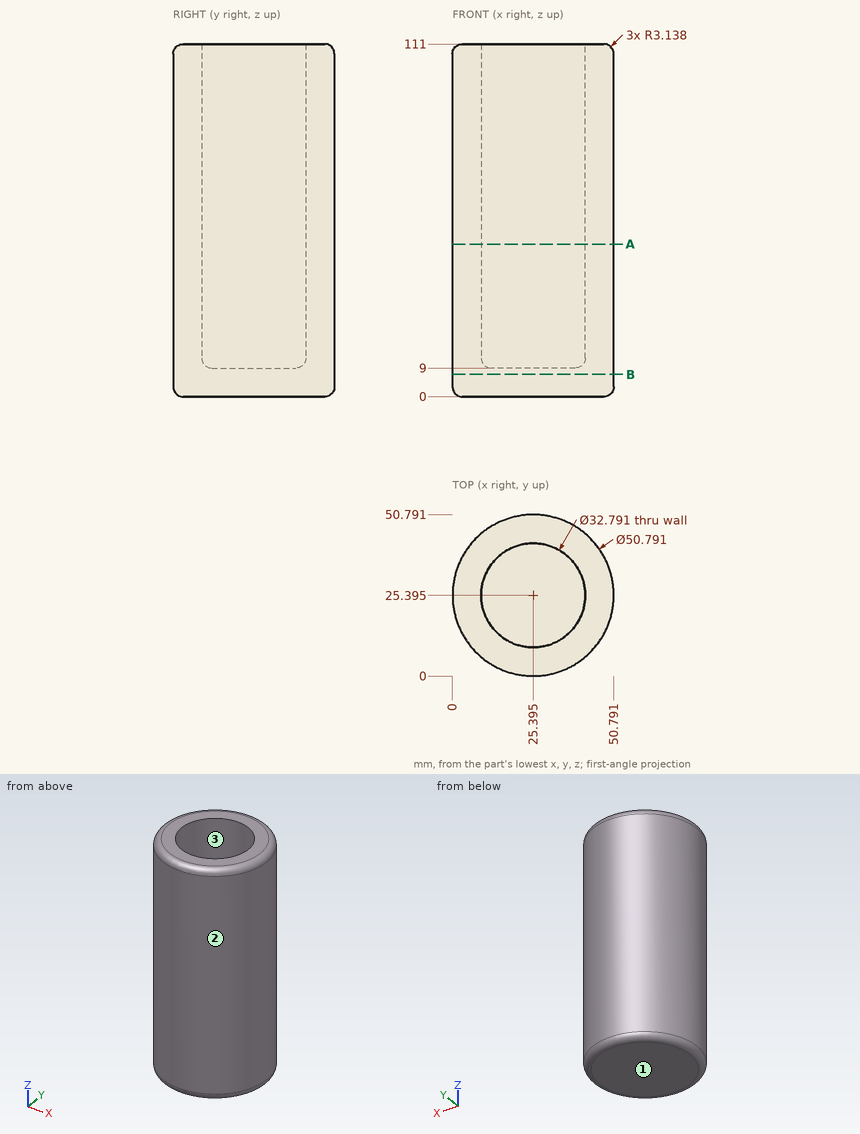
Check sheet for the drawn part. Datum: minimum x, y, z corner. Units: mm. Give positions to 0.01 mm unless a question says otherwise; leave off trailing zeros. Order: outer loops, then holes, each group sorted by start corner. A loop starts at its lowest first (then second) coordinate and runs counter-clockwise, first axis right, second up. Notation, with made-up numbers: (19, 86.25) - (49, 86.25) arc R18 cw to (49, 105.25) - close; hole circle Ø6 at (-10.75, 43.5). An arc over 180 degrees is marked (long way). Answer in a Markdown table with one row per item. Add a question column.
Q1. Material ranges on probe 1 along X at (y, z) = (25, 39.5) (1 decimal); probe 2 along Z at (x, y) = (13.5, 22); probe 3 along X at (y, z) = (32.5, 60) (1 decimal), recorded low to high. Write a range as from..to.
Q2. Cross-section at A-A, the plane z = 48. Enter the section's corners in (x, y) (1 decimal), then the cut area to 3 significant figures.
Q3. Gauge pin test, flat ends, axial feed: pin 1 (1.5 mm diameter, centred on y = 32.5, z = 66, fed in from -X); pin 2 (8 mm diameter, centred on x = 24.5, y = 22, fed in from +Z); pin 3 (4 mm diameter, centred on y = 25, z = 33, fed in from -X); pin 4 (3 mm diameter, centred on y = 45, z = 72.5, fed in from +X) (1 decimal). Record the tip position at first contact, or that the pin passes through.
Q4. Cross-section at B-B, the plane z = 7. Enter the section's corners in (x, y) (1 decimal).
Q5. Mould release check, pull along Y, two halves, no side actions. Record for the marked faces 1, 2 and 3: pulls with the +Y half, pulls with the -Y half, needs draft (parallel to the pull), parting line crosses it, or undercut.
Check values:
| question | item | result |
|---|---|---|
| 1 | probe 1 | x = 0..9, 41.8..50.8 |
| 1 | probe 2 | z = 0..9 |
| 1 | probe 3 | x = 1..10.6, 40.2..49.8 |
| 2 | outline | circle Ø50.8 at (25.4, 25.4); hole circle Ø32.8 at (25.4, 25.4) |
| 2 | area | 1,180 mm^2 |
| 3 | pin 1 | stops at x = 0.81 |
| 3 | pin 2 | stops at z = 9 |
| 3 | pin 3 | stops at x = 0 |
| 3 | pin 4 | stops at x = 43.2 |
| 4 | outline | circle Ø50.8 at (25.4, 25.4) |
| 5 | face 1 | needs draft |
| 5 | face 2 | parting line crosses it |
| 5 | face 3 | undercut |
